For this review, take the finished solid that the model builds, in its own axes (mm). A direction names the side the tool comes from. Coordinates: 2 decimals unless noted, no trailing zeros. Order: outer loops, then holes, each group sorted by start corner. A loop starts at its lowest first (then second) coordinate and runs counter-clockwise, first axis right, second up. Notation, with made-up numbers: (-17.75, 45) -> (-7.75, 45) arc R6 cw to (-7.75, 55) -> close; hole circle Ø1 at (72, 8). An arc over 180 degrees is marked (long way). Return JSON: item names as keys, results as strings. Group by question number.
Item 1: For line 1 along X through (y, z) = (41, 6.75); line 2 along Y through (x, z) = (8, 15.5); line 3 along Z through (x, y) = (44, 10), list the stretches that pass through material, from the lowest coordinate up.
Item 2: Insertion check: pin 1 (7 mm diameter, centred on x = 37.13, y = 40, fed in from +Z); pin 2 (10 mm diameter, centred on y = 11.5, z = 8, fed in from -X); pin 3 (6 mm diameter, centred on y = 11, z = 12.5, fed in from -X); pin 4 (9.5 mm diameter, centred on y = 10, z = 10, fed in from +X). Each pin has a flat end and moves straight along its axis. Give the tip position at first contact, or say it passes through.
Item 3: Draft analysis for pull direction X (two halves, no side actions). For faces 4 (the cylindrical face through (23.89, 2.85, 3.01)), 5 (the cylindrical face through (13.37, 37.41, 9.86)), 6 (the flat face through (10, 6, 13)), state which applies: +X half, -X half, draft (parallel to the pull), parting line (faces both ways), or undercut.
Item 4: Take a section at A-A (y = 40). Write out the cut boundary in (x, z).
Item 5: Machinability: for faces 1 (the flat face through (23, 30, 0)), 2 (the cylindrical face through (4.93, 4.143, 8.699)), 3 (the cylindrical face through (42.06, 4.05, 9.22)), which of the approach directions +Z, -Z, +X, -X, +Y, -Y give a long, thin tool a straight path to every point of the face, cutting with its end or side? Answer none if there is none.
Item 6: Take a section at B-B (z = 7.5). Write out the cut boundary in (x, y), then the cut area to 3 significant figures.
Item 7: Take a section at D-D (y = 11). Write out the cut boundary in (x, z).
```python
from build123d import *

# Parameters (mm, degrees)
SKETCH1_W                      = 47.129705535
SKETCH1_H                      = 50
EXTRUDE1_DEPTH                 = 20
F_8_5_8_5_DIAMETER_HOLE1_D     = 8.5
F_8_5_8_5_DIAMETER_HOLE1_DEPTH = 47.13
F_8_5_8_5_DIAMETER_HOLE1_TIP   = 2.553657631
SKETCH4_R                      = 6
EXTRUDE2_DEPTH                 = 10
EXTRUDE3_START                 = -10
SKETCH3_R                      = 6
EXTRUDE3_DEPTH                 = 10
F_8_5_8_5_DIAMETER_HOLE2_D     = 8.5
FILLET1_R                      = 10


with BuildPart() as part:
    # Sketch1 → Extrude1 (new body)
    with BuildSketch(Plane.XY):
        with Locations((23.564852768, 25)):
            Rectangle(SKETCH1_W, SKETCH1_H)
    extrude(amount=EXTRUDE1_DEPTH)

    # Ø8.5 (8.5) Diameter Hole1
    with Locations(Plane(origin=(47.129705535, 10, 10), x_dir=(0, 0, 1), z_dir=(1, 0, 0))):
        with Locations((0, 0)):
            Hole(F_8_5_8_5_DIAMETER_HOLE1_D / 2, depth=F_8_5_8_5_DIAMETER_HOLE1_DEPTH)
            with Locations((0, 0, -(F_8_5_8_5_DIAMETER_HOLE1_DEPTH + F_8_5_8_5_DIAMETER_HOLE1_TIP / 2))):  # 118° drill point
                Cone(0, F_8_5_8_5_DIAMETER_HOLE1_D / 2, F_8_5_8_5_DIAMETER_HOLE1_TIP, mode=Mode.SUBTRACT)

    # Sketch4 → Extrude2 (cut)
    with BuildSketch(Plane.ZY):
        with Locations((10, 10)):
            Circle(SKETCH4_R)
    extrude(amount=-EXTRUDE2_DEPTH, mode=Mode.SUBTRACT)

    # Sketch3 → Extrude3 (cut)
    with BuildSketch(Plane(origin=(47.129705535, 0, 0), x_dir=(0, 0, -1), z_dir=(1, 0, 0)).offset(EXTRUDE3_START)):
        with Locations(Location((-10, 10, 0), (0, 0, 180))):
            Circle(SKETCH3_R)
    extrude(amount=EXTRUDE3_DEPTH, mode=Mode.SUBTRACT)

    # Ø8.5 (8.5) Diameter Hole2 (through all)
    with Locations(Plane(origin=(37.129705535, 40, 20), x_dir=(1, 0, 0), z_dir=(0, 0, 1))):
        with Locations((0, 0), (-27.129705535, 0)):
            Hole(F_8_5_8_5_DIAMETER_HOLE2_D / 2)

    # Fillet1
    fillet1_edges = [part.edges().sort_by_distance(p)[0] for p in [
        (23.564852768, 0, 20),
        (23.564852768, 0, 0),
    ]]
    fillet(fillet1_edges, radius=FILLET1_R - 0.0001)  # a hair under: the kernel refuses the full size


solid = part.part
```
Findings below:
{
 "1": {"line 1": "x = 0 to 5.87, 14.13 to 33, 41.26 to 47.13", "line 2": "y = 1.65 to 7.6, 12.4 to 36.25, 43.75 to 50", "line 3": "z = 0 to 4, 16 to 20"},
 "2": {"pin 1": "passes through", "pin 2": "stops at x = 0", "pin 3": "stops at x = 10", "pin 4": "stops at x = 37.13"},
 "3": {"face 4": "draft", "face 5": "undercut", "face 6": "-X half"},
 "4": {"outline": "(0, 0) -> (5.75, 0) -> (5.75, 20) -> (0, 20) -> close; (14.25, 0) -> (32.88, 0) -> (32.88, 20) -> (14.25, 20) -> close; (41.38, 0) -> (47.13, 0) -> (47.13, 20) -> (41.38, 20) -> close"},
 "5": {"face 1": "-Z, +X, -X, +Y, -Y", "face 2": "-X", "face 3": "+X"},
 "6": {"outline": "(0, 0.32) -> (47.13, 0.32) -> (47.13, 4.55) -> (37.13, 4.55) -> (37.13, 6.56) -> (10, 6.56) -> (10, 4.55) -> (0, 4.55) -> close; (0, 15.45) -> (10, 15.45) -> (10, 13.44) -> (37.13, 13.44) -> (37.13, 15.45) -> (47.13, 15.45) -> (47.13, 50) -> (0, 50) -> close; hole circle Ø8.5 at (10, 40); hole circle Ø8.5 at (37.13, 40)", "area": "1,820 mm2"},
 "7": {"outline": "(0, 0) -> (47.13, 0) -> (47.13, 4.08) -> (37.13, 4.08) -> (37.13, 5.87) -> (10, 5.87) -> (10, 4.08) -> (0, 4.08) -> close; (0, 15.92) -> (10, 15.92) -> (10, 14.13) -> (37.13, 14.13) -> (37.13, 15.92) -> (47.13, 15.92) -> (47.13, 20) -> (0, 20) -> close"}
}
